For this review, take the finished solid that the model builds, in its own axes (mm). Face numbers are marked on the shaded views. A direction names the side the tool comes from. Coordinates: 2 decimals unless noted, no trailing zeros. Order: outer loops, then holes, each group sorted by start corner. A loop starts at its lowest first (then second) coordinate and runs counter-clockwise, first axis right, second up. Notation, with made-up numbers: M 18,68.25 L 64,68.25 A12 ccw 64,79.25 Z; hole C 85.25,-31 d7. An arc over 180 degrees is marked long. Use CSV: the item, a comma, the result in double quotes.
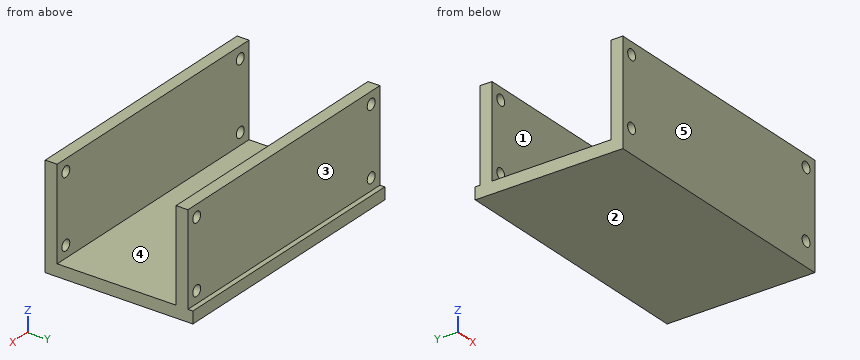
```python
from build123d import *

# Parameters (mm, degrees)
SKETCH1_W           = 66
SKETCH1_H           = 23
SKETCH1_R           = 1.35
BOSS_EXTRUDE1_DEPTH = 3
SKETCH2_W           = 66
SKETCH2_H           = 37.236421537
BOSS_EXTRUDE2_DEPTH = 3


with BuildPart() as part:
    # Sketch1 → Boss-Extrude1 (new body)
    with BuildSketch(Plane(origin=(0, 0, 0), x_dir=(1, 0, 0), z_dir=(0, 1, 0))):
        Rectangle(SKETCH1_W, SKETCH1_H)
        with Locations(Location((-30, -8.5, 0), (0, 0, 270))):
            Circle(SKETCH1_R, mode=Mode.SUBTRACT)
        with Locations(Location((-30, 8.5, 0), (0, 0, 270))):
            Circle(SKETCH1_R, mode=Mode.SUBTRACT)
        with Locations(Location((30, -8.5, 0), (0, 0, 90))):
            Circle(SKETCH1_R, mode=Mode.SUBTRACT)
        with Locations(Location((30, 8.5, 0), (0, 0, 90))):
            Circle(SKETCH1_R, mode=Mode.SUBTRACT)
    boss_extrude1 = extrude(amount=BOSS_EXTRUDE1_DEPTH)

    # Sketch2 → Boss-Extrude2 (add)
    with BuildSketch(Plane(origin=(0, 0, -11.5), x_dir=(-1, 0, 0), z_dir=(0, 0, -1))):
        with Locations((0, 18.618210769)):
            Rectangle(SKETCH2_W, SKETCH2_H)
    extrude(amount=BOSS_EXTRUDE2_DEPTH)

    # Mirror2: Boss-Extrude1 across plane
    add(boss_extrude1.mirror(Plane.ZX.offset(18)))


solid = part.part
```
Item 1: For the marked faces 4 and 5, list the 3-axis set-ups (+Z, -Z, +X, -X, +Y, -Y) from which the entire face can be reached by the end or side of a thin tool; tool diameter is ignored.
Solutions:
face 4,"+Z, +X, -X"
face 5,"+Z, -Z, +X, -X, -Y"
Item 2: Add section A-A on x = 30. State the section outline as (y, z) points, and give its area (3 significant figures).
Solutions:
outline,"M 0,-14.5 L 37.24,-14.5 L 37.24,-11.5 L 36,-11.5 L 36,-9.85 L 33,-9.85 L 33,-11.5 L 3,-11.5 L 3,-9.85 L 0,-9.85 Z; M 0,-7.15 L 3,-7.15 L 3,7.15 L 0,7.15 Z; M 0,9.85 L 3,9.85 L 3,11.5 L 0,11.5 Z; M 33,-7.15 L 36,-7.15 L 36,7.15 L 33,7.15 Z; M 33,9.85 L 36,9.85 L 36,11.5 L 33,11.5 Z"
area,"217 mm^2"
Item 3: To check wall thickness, follow line 1 along X through (y, z) = (1.85, -8.5); line 2 along Z through (x, y) = (30, 1.2); line 3 along Y through (x, z) = (-15.5, -8.25). State the ranges of each line that lie inside material, in increasing order. Write a range as [from, to].
Solutions:
line 1,"[-33, -31.35], [-28.65, 28.65], [31.35, 33]"
line 2,"[-14.5, -9.85], [-7.15, 7.15], [9.85, 11.5]"
line 3,"[0, 3], [33, 36]"
Item 4: Draft analysis for pull direction Y (two halves, no side actions). For the marked faces 1, 2 and 3, state which applies: released by +Y, released by -Y, zero draft, split by the parting line, or undercut.
Solutions:
face 1,"undercut"
face 2,"zero draft"
face 3,"released by +Y"
Item 5: Add section D-D on x = 0. State the section outline as (y, z) points, and give its area (3 significant figures).
Solutions:
outline,"M 0,-14.5 L 37.24,-14.5 L 37.24,-11.5 L 36,-11.5 L 36,11.5 L 33,11.5 L 33,-11.5 L 3,-11.5 L 3,11.5 L 0,11.5 Z"
area,"250 mm^2"
Item 6: Add section C-C on z = -2.5. State the section outline as (x, y) points, and give its area (3 significant figures).
Solutions:
outline,"M -33,0 L 33,0 L 33,3 L -33,3 Z; M -33,33 L 33,33 L 33,36 L -33,36 Z"
area,"396 mm^2"
Item 7: Clearance check with flat-ended pins moving along their axes: pin 1 Ø3.5 at (x, z) = (30, -8.5) entering from +Y; pin 2 Ø5 at (x, y) = (22.5, 13) entering from +Z. State where each tip first meets the part, or that it passes through.
Solutions:
pin 1,"y = 36"
pin 2,"z = -11.5"
Item 8: Add section B-B on z = 8.5. State the section outline as (x, y) points.
Solutions:
outline,"M -33,0 L -31.35,0 L -31.35,3 L -33,3 Z; M -33,33 L -31.35,33 L -31.35,36 L -33,36 Z; M -28.65,0 L 28.65,0 L 28.65,3 L -28.65,3 Z; M -28.65,33 L 28.65,33 L 28.65,36 L -28.65,36 Z; M 31.35,0 L 33,0 L 33,3 L 31.35,3 Z; M 31.35,33 L 33,33 L 33,36 L 31.35,36 Z"
